Verification items for the finished model (mm, model axes). A direction names the side the tool comes from. Coordinates: 2 decimals unless noted, no trailing zeros. Write each loop counter-clockwise with the first axis right and the second up, starting at its lowest first coordinate (ties: lowest second). Pieces come first, ordered by that corner, then holes. Notation, with made-up numbers: (-24.5, -38) -> (1.5, -38) arc R30 cw to (1.5, 1) -> close; hole circle Ø11 at (45, 7.25). An arc over 180 degrees is marked (long way). Use a Markdown table: item, result. Add a question column.
from build123d import *

# Parameters (mm, degrees)
PAD001004_DEPTH    = 2.5
SKETCH006_R        = 2
POCKET003_DEPTH    = 5.001
POCKET003003_DEPTH = 3


with BuildPart() as part:
    # Sketch005 → Pad001004 (new body, symmetric)
    with BuildSketch(Plane.YZ):
        with BuildLine():
            Line((-5, 0), (-7, 0))
            Line((-7, 0), (-7, -5))
            Line((-7, -5), (1.8e-05, -5))
            ThreePointArc((1.8e-05, -5), (3.535528, 3.53554), (-5, 0))
        make_face()
    extrude(amount=PAD001004_DEPTH, both=True)

    # Sketch006 → Pocket003 (cut, through all)
    with BuildSketch(Plane.YZ.offset(2.5)):
        Circle(SKETCH006_R)
    extrude(amount=-POCKET003_DEPTH, mode=Mode.SUBTRACT)

    # Sketch007 → Pocket003003 (cut)
    with BuildSketch(Plane.YZ.offset(2.5)):
        Polygon((-3.059956, 0), (-1.529978, 2.65), (1.529978, 2.65), (3.059956, 0), (1.529978, -2.65), (-1.529978, -2.65), align=None)
    extrude(amount=-POCKET003003_DEPTH, mode=Mode.SUBTRACT)


solid = part.part
1) Cross-section at D-D on y = 4. Record the boundary of the cut face in (x, z), then the cut area to 3 significant figures.
2) Gauge pin test, flat ends, axial feed: pin 1 (2.5 mm diameter, centred on x = 1, y = -0.5, fed in from +Z); pin 2 (4.5 mm diameter, centred on y = 0, z = 0, fed in from +X); pin 3 (0.6 mm diameter, centred on x = 0, y = -5.5, fed in from +Z); pin 4 (2 mm diameter, centred on x = 2, z = 3, fed in from -Y). Record the tip position at first contact, or that the pin passes through.
3) Cross-section at A-A on x = 1.3. Record the boundary of the cut face in (y, z).
4) Cross-section at B-B on z = -0.25. Record the boundary of the cut face in (x, y), then the cut area to 3 significant figures.
5) Cross-section at C-C on y = 1.75. Record the boundary of the cut face in (x, z), then the cut area to 3 significant figures.
6) Thickness scan on L1, parallel to Z at x = -1.65, y = 0; L2, parallel to Z at x = -0.15, y = -5.25; L3, parallel to Y at x = -0.25, z = 0.75. Record the ranges inside material, lowest first.
7) Release check for a two-part mould opening along Y. For faces 3 (the face through (0, -6, 0)), 4 (the face through (0, -7, -2)), 5 (the face through (1, 0, 2.65)), 6 (the face through (1.021, 2.284, 1.344)) record: released by +Y, released by -Y, zero draft, split by the parting line, or undercut.
8) Set-up check for faces 1 (the face through (1, 0, -2.65)), 2 (the face through (0, 4, 3)): record each of +Z, -Z, +X, -X, +Y, -Y from which the full face is reachable in a straight line by a thin tool's end or side.
Returned:
| question | item | result |
|---|---|---|
| 1 | outline | (-2.5, -3) -> (2.5, -3) -> (2.5, 3) -> (-2.5, 3) -> close |
| 1 | area | 30.0 mm² |
| 2 | pin 1 | stops at z = 5 |
| 2 | pin 2 | stops at x = -0.5 |
| 2 | pin 3 | stops at z = 0 |
| 2 | pin 4 | stops at y = -4.58 |
| 3 | outline | (-7, -5) -> (0, -5) arc R5 ccw (long way) to (-5, 0) -> (-7, 0) -> close; hole (-3.06, 0) -> (-1.53, -2.65) -> (1.53, -2.65) -> (3.06, 0) -> (1.53, 2.65) -> (-1.53, 2.65) -> close |
| 4 | outline | (-2.5, -7) -> (2.5, -7) -> (2.5, -2.92) -> (-0.5, -2.92) -> (-0.5, -1.98) -> (-2.5, -1.98) -> close; (-2.5, 1.98) -> (-0.5, 1.98) -> (-0.5, 2.92) -> (2.5, 2.92) -> (2.5, 4.99) -> (-2.5, 4.99) -> close |
| 4 | area | 34.5 mm² |
| 5 | outline | (-2.5, -4.68) -> (2.5, -4.68) -> (2.5, -2.27) -> (-0.5, -2.27) -> (-0.5, -0.97) -> (-2.5, -0.97) -> close; (-2.5, 0.97) -> (-0.5, 0.97) -> (-0.5, 2.27) -> (2.5, 2.27) -> (2.5, 4.68) -> (-2.5, 4.68) -> close |
| 5 | area | 29.4 mm² |
| 6 | L1 | z = -5 to -2, 2 to 5 |
| 6 | L2 | z = -5 to 0 |
| 6 | L3 | y = -4.94 to -2.63, 2.63 to 4.94 |
| 7 | face 3 | zero draft |
| 7 | face 4 | released by -Y |
| 7 | face 5 | undercut |
| 7 | face 6 | undercut |
| 8 | face 1 | +X |
| 8 | face 2 | +X, -X |
